Build history of the part. All positions in model axes, mm. Face numbers are marked on the shaded views. Give positions to 0.01 mm unless a question says otherwise; leave off trailing zeros. Loops run counter-clockwise (first coordinate to the right, second up) from the corner with the lowest first, then second, coordinate; pieces in that order, holes last. Notation, with made-up numbers: (-38, 43) -> (10, 43) arc R19 cw to (10, 48) -> close; hole circle Ø2 at (-18.5, 84). An arc over 180 degrees is marked (long way). Answer as a JSON object with one key per item and string values. Group by question number.
from build123d import *

# Parameters (mm, degrees)
SKETCH1_R           = 67.31
SKETCH1_R_2         = 66.04
BOSS_EXTRUDE1_DEPTH = 457.2
SKETCH3_W           = 6.35
SKETCH3_H           = 203.2
CUT_EXTRUDE1_DEPTH  = 68.31
CIRPATTERN1_COUNT   = 4


with BuildPart() as part:
    # Sketch1 → Boss-Extrude1 (new body)
    with BuildSketch(Plane(origin=(0, 0, 0), x_dir=(1, 0, 0), z_dir=(0, 1, 0))):
        Circle(SKETCH1_R)
        Circle(SKETCH1_R_2, mode=Mode.SUBTRACT)
    extrude(amount=BOSS_EXTRUDE1_DEPTH)

    # Sketch3 → Cut-Extrude1 (cut, symmetric)
    with BuildSketch(Plane.XY):
        with Locations((0, 152.4)):
            Rectangle(SKETCH3_W, SKETCH3_H)
    cut_extrude1 = extrude(amount=CUT_EXTRUDE1_DEPTH, both=True, mode=Mode.SUBTRACT)

    # CirPattern1: Cut-Extrude1 ×4 about axis
    cirpattern1_axis = Axis((0, 0, 0), (0, 1, 0))
    for i in range(1, CIRPATTERN1_COUNT):
        add(cut_extrude1.rotate(cirpattern1_axis, i * 360 / CIRPATTERN1_COUNT), mode=Mode.SUBTRACT)


solid = part.part
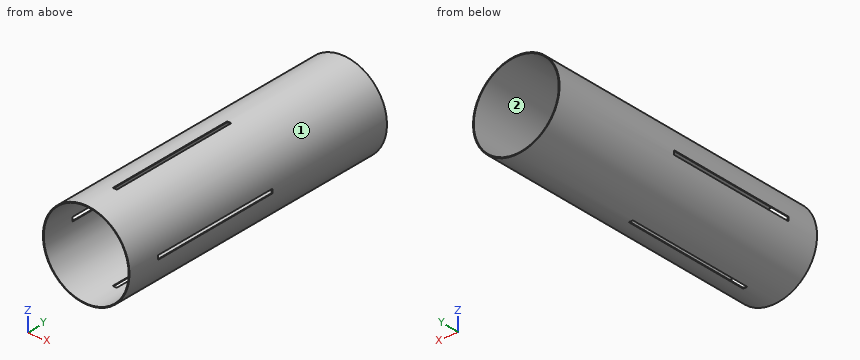
(1) Saw through at A-A on x = 29.5. List the corners of the cut face in (y, z), plus the area to 3 significant figures.
(2) Saw through at C-C on z = 8.5. List the corners of the cut face in (x, y), plus the area to 3 significant figures.
(3) Saw through at B-B on y = 163. List the corners of the cut face in (x, z) (3 decimals).
(4) Pin check, flat tips, straight feed: pin 1 (2 mm diameter, centred on x = -5.5, y = 202.5, fed in from +Z); pin 2 (10 mm diameter, centred on y = 181.5, z = 2, fed in from +X); pin 3 (8 mm diameter, centred on y = 395, z = -30, fed in from -X). Stop position of each tip, or through.
(5) Pull direction X, two halves, no side cores. Call the marked faces 1 and 2: pulls with the +X half, pulls with the -X half, needs draft (parallel to the pull), parting line crosses it, or undercut.
(6) Saw through at D-D on y = 425. List the corners of the cut face in (x, z).
(7) Probe line 1 along X through (y, z) = (296.5, 0); line 2 along Z through (x, y) = (-28.5, 200). List the from-to ranges inside material, lowest first. Write a range as [from, to].
Calculated:
{
 "1": {"outline": "(0, -60.5) -> (457.2, -60.5) -> (457.2, -59.08) -> (0, -59.08) -> close; (0, 59.08) -> (457.2, 59.08) -> (457.2, 60.5) -> (0, 60.5) -> close", "area": "1,290 mm^2"},
 "2": {"outline": "(-66.77, 0) -> (-65.49, 0) -> (-65.49, 457.2) -> (-66.77, 457.2) -> close; (65.49, 0) -> (66.77, 0) -> (66.77, 457.2) -> (65.49, 457.2) -> close", "area": "1,170 mm^2"},
 "3": {"outline": "(-67.235, -3.175) arc R67.31 ccw to (-3.175, -67.235) -> (-3.175, -65.964) arc R66.04 cw to (-65.964, -3.175) -> close; (-67.235, 3.175) -> (-65.964, 3.175) arc R66.04 cw to (-3.175, 65.964) -> (-3.175, 67.235) arc R67.31 ccw to start; (3.175, -67.235) arc R67.31 ccw to (67.235, -3.175) -> (65.964, -3.175) arc R66.04 cw to (3.175, -65.964) -> close; (3.175, 65.964) arc R66.04 cw to (65.964, 3.175) -> (67.235, 3.175) arc R67.31 ccw to (3.175, 67.235) -> close"},
 "4": {"pin 1": "stops at z = 67.16", "pin 2": "stops at x = 67.24", "pin 3": "stops at x = -62.09"},
 "5": {"face 1": "parting line crosses it", "face 2": "undercut"},
 "6": {"outline": "circle Ø134.62 at (0, 0); hole circle Ø132.08 at (0, 0)"},
 "7": {"line 1": "x = [-67.31, -66.04], [66.04, 67.31]", "line 2": "z = [-60.98, -59.57], [59.57, 60.98]"}
}
